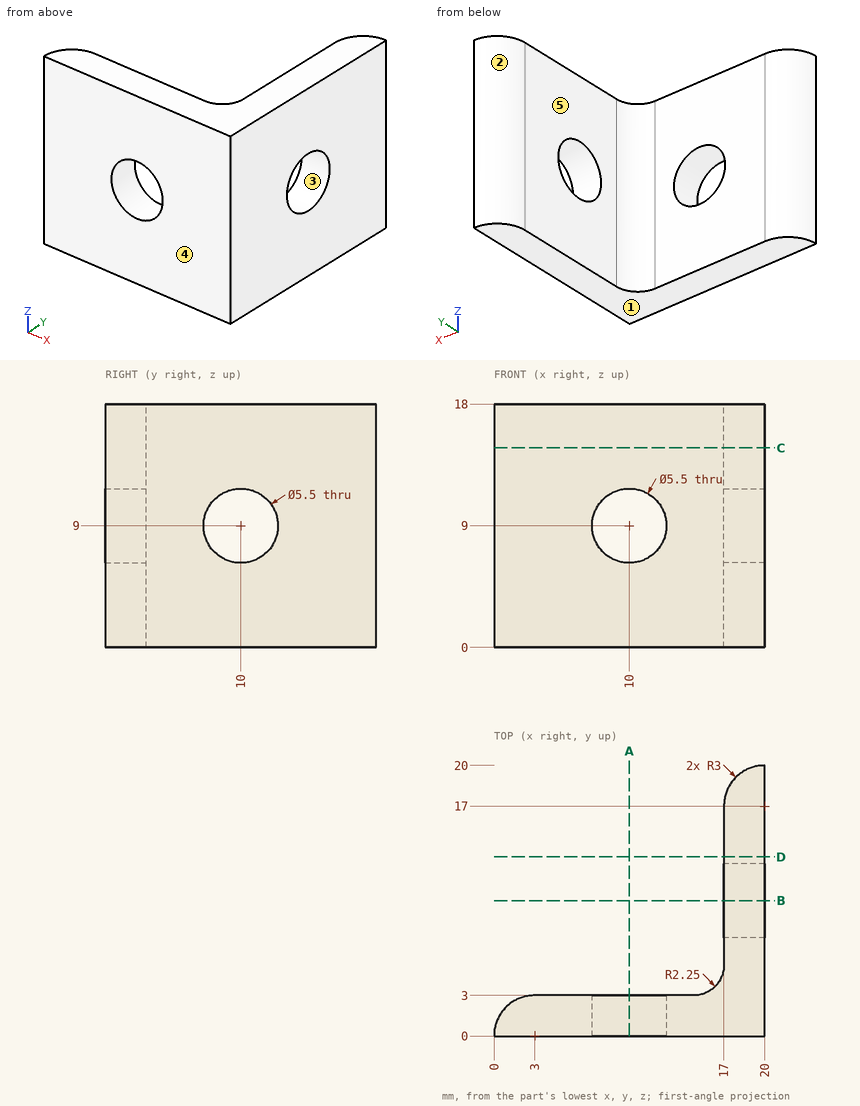
Input: dimensioned drawing with shaded views. Units: mm. Origin: part minimum x, y, z. A direction names the side the tool comes from. Give positions to 0.01 mm unless a question says otherwise; leave off trailing zeros. Loops run counter-clockwise (first coordinate to the right, second up) from the corner with the lowest first, then second, coordinate; pieces in that order, holes last. Notation, with made-up numbers: M 10,23 L 26,23 A19 cw 26,41 Z; hole C 77,40.25 d2. An arc over 180 degrees is marked long. Put each result on its own line as item: value. Start each with the question number.
1) Pull-direction query (Z, two-part tool) for the marked faces 1, 2 and 3; classes: pulls with the +Z half, pulls with the -Z half, needs draft (parallel to the pull), parting line crosses it, or undercut.
2) Contact query for flat-ended pins moving along their axis: pin 1 (2 mm diameter, centred on y = 7.5, z = 11.5, fed in from -X); pin 2 (3.5 mm diameter, centred on x = 10.5, z = 13, fed in from +Y); pin 3 (4 mm diameter, centred on x = 13.5, y = 15, fed in from +Z); pin 4 (1 mm diameter, centred on x = 17, z = 15, fed in from +Y). Output: stop coordinate, or through.
3) Ray query, line 1 along Z through (x, y) = (10, 0.65); line 2 along Y through (x, z) = (7, 14.25); line 3 along Y through (x, z) = (18.95, 9). Return the intervals inside material, ascending.
4) Access query for the marked faces 4 and 5. Directions: +Z, -Z, +X, -X, +Y, -Y. A direction counts if a zero-diameter tool reaches every point of the face in a straight line with its end or side. Return the directions, or none.
5) Cut plane D-D (y = 13.25). Output: boundary loops of the cut face in (x, z), then the cut area to 3 significant figures.
6) Cut plane C-C (z = 14.75). Output: boundary loops of the cut face in (x, y).
7) Cut plane A-A (x = 10). Output: boundary loops of the cut face in (y, z).
8) Cut plane B-B (y = 10). Output: boundary loops of the cut face in (x, z).
Verdict:
1. face 1: pulls with the -Z half
1. face 2: needs draft
1. face 3: undercut
2. pin 1: x = 17
2. pin 2: y = 3
2. pin 3: through
2. pin 4: y = 18.66
3. line 1: 0 to 6.25, 11.75 to 18
3. line 2: 0 to 3
3. line 3: 0 to 7.25, 12.75 to 19.81
4. face 4: +Z, -Z, +X, -X, -Y
4. face 5: +Z, -Z, -X, +Y
5. outline: M 17,0 L 20,0 L 20,18 L 17,18 Z
5. area: 54.0 mm2
6. outline: M 0,0 L 20,0 L 20,20 A3 ccw 17,17 L 17,5.25 A2.25 cw 14.75,3 L 3,3 A3 ccw Z
7. outline: M 0,0 L 3,0 L 3,6.25 L 0,6.25 Z; M 0,11.75 L 3,11.75 L 3,18 L 0,18 Z
8. outline: M 17,0 L 20,0 L 20,6.25 L 17,6.25 Z; M 17,11.75 L 20,11.75 L 20,18 L 17,18 Z
